Build history of the part. All positions in model axes, mm. Face numbers are marked on the shaded views. Round coordinates to 2 decimals unless told otherwise and drop trailing zeros. Order: outer loops, then holes, each group sorted by start corner. A loop starts at its lowest first (then second) coordinate and runs counter-clockwise, first axis right, second up. Notation, with made-up numbers: (-16, 60.5) -> (23, 60.5) arc R26 ccw to (23, 82.5) -> close; hole circle Ø5 at (-9.75, 11). An arc over 180 degrees is marked (long way). Use a Markdown table: item, result. Add a question column.
Item 1: Slice it at D-D, the plane z = 342.5. Give the cut face in (x, y), plus the area to 3 significant figures.
Item 2: Probe L1, parallel to X at y = -85, z = 387; L2, parallel to Y at x = -62, z = 349.5; L3, parallel to Y at x = 46, z = 204.5. List the from-to ranges inside material, lowest first.
Item 3: Pin check, flat tips, straight feed: pin 1 (1 mm diameter, centred on x = -4, y = -61.5, fed in from -Z); pin 2 (1.5 mm diameter, centred on x = -22, y = -68, fed in from -Z). Stop position of each tip, or through.
Item 4: Two-plate mould, pull along Y, no slides. Class the marked faces 1, 2, 3 and 4: released by +Y, released by -Y, zero draft, split by the parting line, or undercut.
Item 5: Slice it at A-A, the plane z = 200. Give the cut face in (x, y), plus the area to 3 significant figures.
Item 6: Slice it at B-B, the plane x = -24.5. Give the cut face in (y, z), plus the area to 3 significant figures.
Item 7: Slice it at C-C, the plane y = -91. Give the cut face in (x, z), plus the area to 3 significant figures.
from build123d import *

# Parameters (mm, degrees)
BOSS_EXTRUDE1_DEPTH      = 63.5
BOSS_EXTRUDE1_DEPTH_BACK = 63.5
BOSS_EXTRUDE2_DEPTH      = 4.826


with BuildPart() as part:
    # Sketch1 → Boss-Extrude1 (new, two sides: drawn at the far end of the back side and taken through both)
    with BuildSketch(Plane(origin=(0, 0, 0), x_dir=(0, 0, -1), z_dir=(1, 0, 0)).offset(-BOSS_EXTRUDE1_DEPTH_BACK)):
        with BuildLine():
            Line((0, -114.3), (-381, -114.3))
            ThreePointArc((-381, -114.3), (-412.045495931, -69.85), (-381, -25.4))
            Line((-381, -25.4), (0, 114.3))
            Line((0, 114.3), (0, 119.126))
            Line((0, 119.126), (-1.661372937, 118.8310171))
            Line((-1.661372937, 118.8310171), (-382.661372937, -20.8689829))
            ThreePointArc((-382.661372937, -20.8689829), (-416.86965301, -70.288504669), (-381.835461036, -119.126))
            Line((-381.835461036, -119.126), (0, -119.126))
            Line((0, -119.126), (0, -114.3))
        make_face()
    extrude(amount=BOSS_EXTRUDE1_DEPTH + BOSS_EXTRUDE1_DEPTH_BACK)

    # Sketch2 → Boss-Extrude2 (add)
    with BuildSketch(Plane(origin=(63.5, 0, 0), x_dir=(0, 0, -1), z_dir=(1, 0, 0))):
        with BuildLine():
            Line((-381.835461036, -119.126), (0, -119.126))
            Line((0, -119.126), (0, 119.126))
            Line((0, 119.126), (-1.661372937, 118.8310171))
            Line((-1.661372937, 118.8310171), (-382.661372937, -20.8689829))
            ThreePointArc((-382.661372937, -20.8689829), (-416.86965301, -70.288504669), (-381.835461036, -119.126))
        make_face()
    boss_extrude2 = extrude(amount=BOSS_EXTRUDE2_DEPTH)

    # Mirror1: Boss-Extrude2 across plane
    add(boss_extrude2.mirror(Plane(origin=(0, 0, 0), x_dir=(0, 0, 1), z_dir=(1, 0, 0))))


solid = part.part
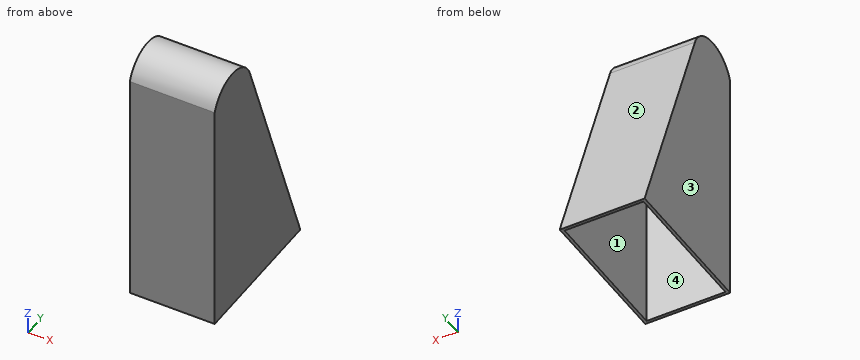
Check sheet entries:
| question | item | result |
|---|---|---|
| 1 | outline | (-68.33, -119.13) -> (68.33, -119.13) -> (68.33, -6.14) -> (-68.33, -6.14) -> close; hole (-63.5, -114.3) -> (63.5, -114.3) -> (63.5, -11.28) -> (-63.5, -11.28) -> close |
| 1 | area | 2,360 mm2 |
| 2 | L1 | -68.33 to -63.5, 63.5 to 68.33 |
| 2 | L2 | -119.13 to -114.3, -13.85 to -8.71 |
| 2 | L3 | -119.13 to -114.3, 39.32 to 44.46 |
| 3 | pin 1 | z = 411.21 |
| 3 | pin 2 | z = 411.97 |
| 4 | face 1 | undercut |
| 4 | face 2 | released by +Y |
| 4 | face 3 | zero draft |
| 4 | face 4 | undercut |
| 5 | outline | (-68.33, -119.13) -> (68.33, -119.13) -> (68.33, 46.11) -> (-68.33, 46.11) -> close; hole (-63.5, -114.3) -> (63.5, -114.3) -> (63.5, 40.97) -> (-63.5, 40.97) -> close |
| 5 | area | 2,860 mm2 |
| 6 | outline | (-119.13, 0) -> (-114.3, 0) -> (-114.3, 381) arc R47.34 cw to (-25.4, 381) -> (114.3, 0) -> (119.13, 0) -> (118.83, 1.66) -> (-20.87, 382.66) arc R52.17 ccw to (-119.13, 381.84) -> close |
| 6 | area | 4,390 mm2 |
| 7 | outline | (-68.33, 0) -> (-63.5, 0) -> (-63.5, 407.06) -> (63.5, 407.06) -> (63.5, 0) -> (68.33, 0) -> (68.33, 412.39) -> (-68.33, 412.39) -> close |
| 7 | area | 4,660 mm2 |
